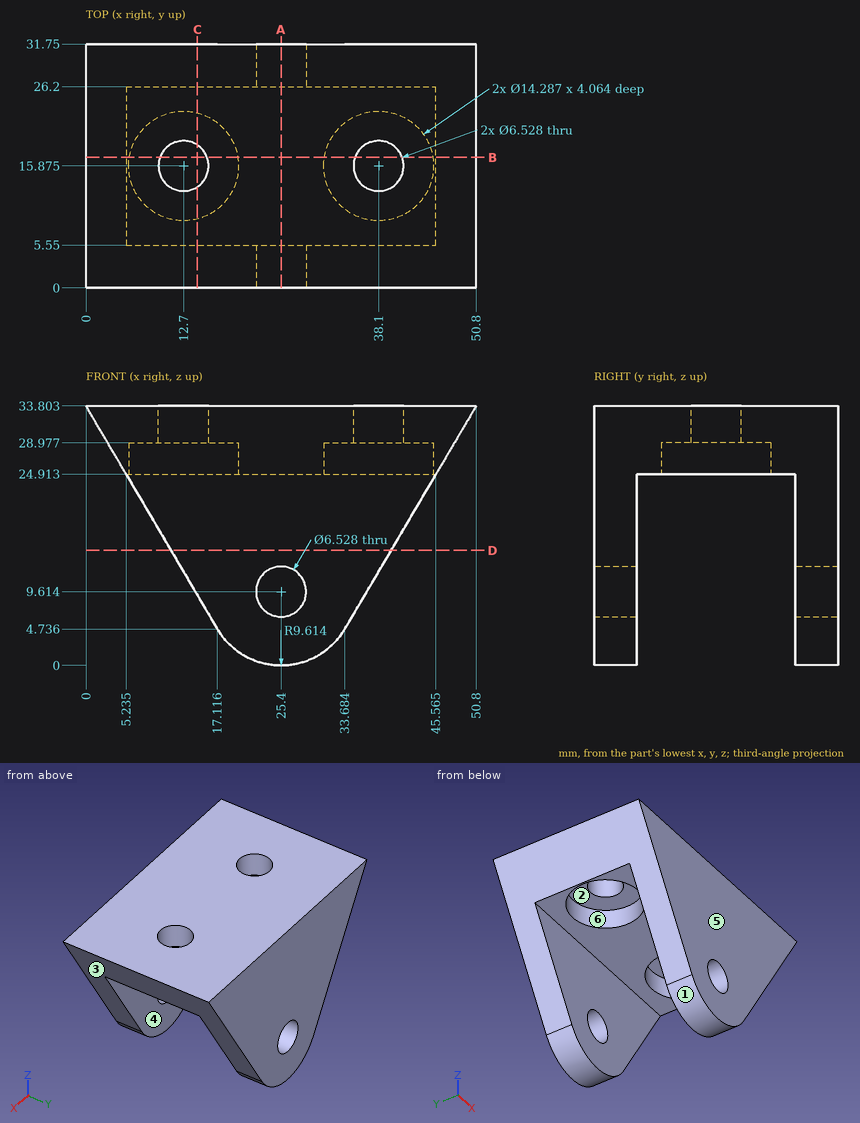
Geometry: see drawing. Coordinates: mm, zero at the bounding-box minimum. A direction names the side the tool comes from. Give positions to 0.01 mm unless a question says otherwise; leave off trailing zeros. Loops run counter-clockwise (first coordinate to the right, second up) from the corner with the lowest first, then second, coordinate; pieces in that order, holes last. Notation, with made-up numbers: (-29, 56.5) -> (-24, 56.5) arc R19 cw to (-24, 73.5) -> close; hole circle Ø10 at (49.5, -4). An arc over 180 degrees is marked (long way). Use one line per item in the form item = value.
Item 1: Pin query (flat end, axial travel): P1, Ø4.5, axis at x = 16, y = 15, coming from the -Z side; P2, Ø4, axis at y = 22.5, z = 15, coming from the +X side; P3, Ø7.5, axis at x = 25.4, z = 9.61, coming from the -Y side; P4, Ø11.5, axis at x = 39, y = 13, coming from the -Z side. Return the tip coordinate at first contact, or that it passes through.
A:
P1 = 28.98
P2 = through
P3 = 0
P4 = 24.91
Item 2: Access query for the marked faces 4, 5 and 6. Directions: +Z, -Z, +X, -X, +Y, -Y. A direction counts if a zero-diameter tool reaches every point of the face in a straight line with its end or side. Return the directions, or none.
A:
face_4 = -Z, +X, -X
face_5 = +Z, -Z, +X, -X, -Y
face_6 = -Z
Item 3: Draft query along X for the marked faces 1, 2 and 3. Return one class per face: pulls with the +X half, pulls with the -X half, needs draft (parallel to the pull), parting line crosses it, or undercut.
A:
face_1 = parting line crosses it
face_2 = undercut
face_3 = pulls with the +X half
Item 4: Section query B-B on y = 17. Output: boundary loops of the cut face in (x, z) (1 decimal).
A:
outline = (0, 33.8) -> (5.2, 24.9) -> (5.6, 24.9) -> (5.6, 29) -> (9.6, 29) -> (9.6, 33.8) -> close; (15.8, 29) -> (19.8, 29) -> (19.8, 24.9) -> (31, 24.9) -> (31, 29) -> (35, 29) -> (35, 33.8) -> (15.8, 33.8) -> close; (41.2, 29) -> (45.2, 29) -> (45.2, 24.9) -> (45.6, 24.9) -> (50.8, 33.8) -> (41.2, 33.8) -> close
Item 5: Line query: probe 1 along Y at (x, z) = (32, 8.5); probe 2 along Y at (x, z) = (38.1, 26.7); probe 3 along X at (y, z) = (30.5, 8) (1 decimal). Output: solid intervals per line, ascending.
A:
probe_1 = 0 to 5.55, 26.2 to 31.75
probe_2 = 0 to 8.73, 23.02 to 31.75
probe_3 = 15.2 to 22.6, 28.2 to 35.6
Item 6: Section query C-C on x = 14.5. Output: boundary loops of the cut face in (y, z).
A:
outline = (0, 9.18) -> (5.55, 9.18) -> (5.55, 24.91) -> (8.96, 24.91) -> (8.96, 28.98) -> (13.15, 28.98) -> (13.15, 33.8) -> (0, 33.8) -> close; (18.6, 28.98) -> (22.79, 28.98) -> (22.79, 24.91) -> (26.2, 24.91) -> (26.2, 9.18) -> (31.75, 9.18) -> (31.75, 33.8) -> (18.6, 33.8) -> close
Item 7: Section query D-D on z = 15. Output: boundary loops of the cut face in (x, y), and give its area (3 significant figures).
A:
outline = (11.07, 0) -> (39.73, 0) -> (39.73, 5.55) -> (11.07, 5.55) -> close; (11.07, 26.2) -> (39.73, 26.2) -> (39.73, 31.75) -> (11.07, 31.75) -> close
area = 318 mm^2
Item 8: Section query A-A on x = 25.4. Output: boundary loops of the cut face in (y, z).
A:
outline = (0, 0) -> (5.55, 0) -> (5.55, 6.35) -> (0, 6.35) -> close; (0, 12.88) -> (5.55, 12.88) -> (5.55, 24.91) -> (26.2, 24.91) -> (26.2, 12.88) -> (31.75, 12.88) -> (31.75, 33.8) -> (0, 33.8) -> close; (26.2, 0) -> (31.75, 0) -> (31.75, 6.35) -> (26.2, 6.35) -> close
